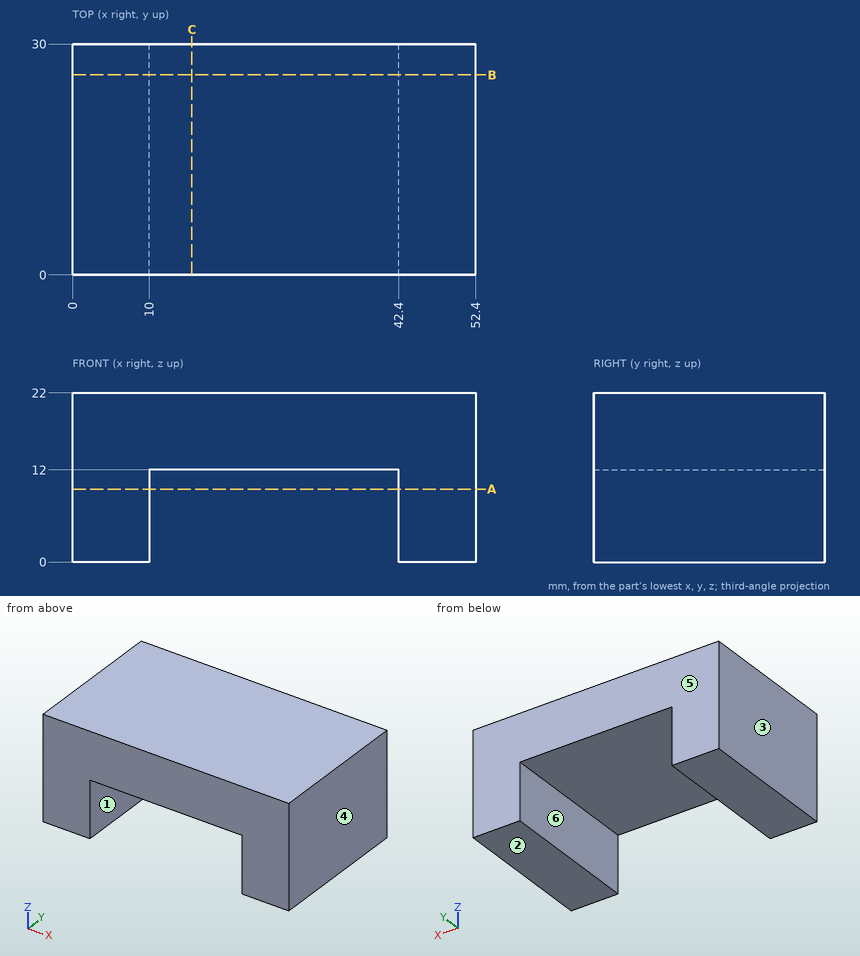
Job drawing, mm, ordinate dimensions from the low corner. One solid piece. A direction names the side the tool comes from. Give positions to 0.01 mm unless a question says otherwise; leave off trailing zeros. Loops run counter-clockwise (first coordinate to the right, second up) from the corner with the lowest first, then second, coordinate; pieces in that order, holes last. Notation, with made-up numbers: M 13.5,-13.75 L 25.5,-13.75 A16 cw 25.5,4.25 Z; hole C 28,-11.75 d11. An arc over 180 degrees is marked long. Answer in a Markdown table with one row per item. Add a question column.
Item 1: Band-saw the part on A-A on z = 9.5. Give the cut face in (x, y).
Item 2: Band-saw the part on C-C on x = 15.5. Give the cut face in (y, z), then the cut area to 3 significant figures.
Item 3: Tool access for the marked faces 5 and 6: list every direction of +Z, -Z, +X, -X, +Y, -Y with a clear straight run to the whole face (end or side of a thin tool).
Item 4: Mould opens along X. For the marked faces 1, 2, 3 and 4 say: +X half, -X half, draft (parallel to the pull), parting line (faces both ways), or undercut.
Item 5: Band-saw the part on B-B on y = 26. Give the cut face in (x, z).
Item 6: Drop flat-ended pins along their axis: P1, Ø12, axis at x = 20, y = 15, coming from the -Z side; P2, Ø8, axis at x = 35, z = 4.5, coming from the +Y side. Give the stop position or say it passes through.
Item 7: Probe probe 1 along X at (y, z) = (10, 2.5); probe 2 along Z at (x, y) = (22.5, 7). List the from-to ranges inside material, lowest first.
Reply:
| question | item | result |
|---|---|---|
| 1 | outline | M 0,0 L 10,0 L 10,30 L 0,30 Z; M 42.4,0 L 52.4,0 L 52.4,30 L 42.4,30 Z |
| 2 | outline | M 0,12 L 30,12 L 30,22 L 0,22 Z |
| 2 | area | 300 mm^2 |
| 3 | face 5 | +Z, -Z, +X, -X, +Y |
| 3 | face 6 | -Z, +Y, -Y |
| 4 | face 1 | undercut |
| 4 | face 2 | draft |
| 4 | face 3 | -X half |
| 4 | face 4 | +X half |
| 5 | outline | M 0,0 L 10,0 L 10,12 L 42.4,12 L 42.4,0 L 52.4,0 L 52.4,22 L 0,22 Z |
| 6 | P1 | stops at z = 12 |
| 6 | P2 | passes through |
| 7 | probe 1 | x = 0 to 10, 42.4 to 52.4 |
| 7 | probe 2 | z = 12 to 22 |
